Check sheet for the modelled part. Datum: model origin and axes. Units: mm. A direction names the side the tool comes from. Round coordinates to 2 decimals unless told otherwise and drop trailing zeros. Order: outer loops, then holes, each group sorted by start corner. A loop starts at its lowest first (then second) coordinate and runs counter-clockwise, first axis right, second up. Notation, with made-up numbers: (32, -6.5) -> (50, -6.5) arc R13 cw to (50, -1.5) -> close; hole circle Ø5 at (-8.5, 6.25). An arc over 180 degrees is marked (long way). Answer in a Markdown table with one row per item.
from build123d import *

# Parameters (mm, degrees)
SKETCH1_R           = 8.9535
SKETCH1_R_2         = 2
BOSS_EXTRUDE1_DEPTH = 1.016
SKETCH2_R           = 6.0325
SKETCH2_R_2         = 2
BOSS_EXTRUDE2_DEPTH = 6.985
SKETCH3_R           = 8.9535
SKETCH3_R_2         = 2
BOSS_EXTRUDE3_DEPTH = 1.016


with BuildPart() as part:
    # Sketch1 → Boss-Extrude1 (new body)
    with BuildSketch(Plane.XY):
        Circle(SKETCH1_R)
        Circle(SKETCH1_R_2, mode=Mode.SUBTRACT)
    extrude(amount=BOSS_EXTRUDE1_DEPTH)

    # Sketch2 → Boss-Extrude2 (add)
    with BuildSketch(Plane.XY.offset(1.016)):
        Circle(SKETCH2_R)
        Circle(SKETCH2_R_2, mode=Mode.SUBTRACT)
    extrude(amount=BOSS_EXTRUDE2_DEPTH)

    # Sketch3 → Boss-Extrude3 (add)
    with BuildSketch(Plane.XY.offset(8.001)):
        Circle(SKETCH3_R)
        Circle(SKETCH3_R_2, mode=Mode.SUBTRACT)
    extrude(amount=BOSS_EXTRUDE3_DEPTH)


solid = part.part
Item 1: Scan lines: line 1 (Z direction, x = -7, y = -4.75); line 2 (Y direction, x = 0, z = 3); line 3 (X direction, y = 0.75, z = 4). Record each from-to range of solid material in increasing order. Write a range as [from, to].
Result sheet:
| item | result |
|---|---|
| line 1 | z = [0, 1.02], [8, 9.02] |
| line 2 | y = [-6.03, -2], [2, 6.03] |
| line 3 | x = [-5.99, -1.85], [1.85, 5.99] |
Item 2: Cross-section at A-A (x = 0). Record the boundary of the cut face in (y, z), and give its area (3 significant figures).
Result sheet:
| item | result |
|---|---|
| outline | (-8.95, 0) -> (-2, 0) -> (-2, 9.02) -> (-8.95, 9.02) -> (-8.95, 8) -> (-6.03, 8) -> (-6.03, 1.02) -> (-8.95, 1.02) -> close; (2, 0) -> (8.95, 0) -> (8.95, 1.02) -> (6.03, 1.02) -> (6.03, 8) -> (8.95, 8) -> (8.95, 9.02) -> (2, 9.02) -> close |
| area | 84.6 mm^2 |
Item 3: Depth check by flat-ended pin: P1, Ø1.5, axis at y = -5, z = 3, coming from the +X side; P2, Ø2, axis at x = -3, z = 5.5, coming from the +Y side; P3, Ø3, axis at x = -0.5, z = 5.5, coming from the -Y side. Enter the tip coordinate at first touch or a pass-through.
Result sheet:
| item | result |
|---|---|
| P1 | stops at x = 4.28 |
| P2 | stops at y = 5.69 |
| P3 | stops at y = -6.03 |
Item 4: Mould release check, pull along Z, two halves, no side actions. Record for faces 1 (the cylindrical face through (-1.94, -8.74, 8.5)), 2 (the flat face through (2, -2, 9.017)), 3 (the flat face through (2, -6, 1.016)): pulls with the +Z half, pulls with the -Z half, needs draft (parallel to the pull), parting line crosses it, or undercut.
Result sheet:
| item | result |
|---|---|
| face 1 | needs draft |
| face 2 | pulls with the +Z half |
| face 3 | undercut |
Item 5: Cross-section at C-C (z = 1.25). Record the boundary of the cut face in (x, y) (1 decimal), and give its area (3 significant figures).
Result sheet:
| item | result |
|---|---|
| outline | circle Ø12.1 at (0, 0); hole circle Ø4 at (0, 0) |
| area | 102 mm^2 |
Item 6: Cross-section at D-D (y = 8). Record the boundary of the cut face in (x, z), and give its area (3 significant figures).
Result sheet:
| item | result |
|---|---|
| outline | (-4.02, 0) -> (4.02, 0) -> (4.02, 1.02) -> (-4.02, 1.02) -> close; (-4.02, 8) -> (4.02, 8) -> (4.02, 9.02) -> (-4.02, 9.02) -> close |
| area | 16.3 mm^2 |
Item 7: Set-up check for faces 4 (the cylindrical face through (0, -2, 4)), 5 (the cylindrical face through (5.754, 1.812, 4.46)): record each of +Z, -Z, +X, -X, +Y, -Y from which the full face is reachable in a straight line by a thin tool's end or side.
Result sheet:
| item | result |
|---|---|
| face 4 | +Z, -Z |
| face 5 | none |
